```python
from build123d import *

# Parameters (mm, degrees)
SKETCH1_R               = 19.05
BOSS_EXTRUDE1_DEPTH     = 12.7
SKETCH2_R               = 3.175
BOSS_EXTRUDE2_DEPTH     = 12.7
CUT_EXTRUDE1_DEPTH      = 30.784140075
CUT_EXTRUDE1_DEPTH_BACK = 30.784140075
SKETCH4_R               = 6.477
SKETCH5_R               = 3.175
CUT_EXTRUDE2_DEPTH      = 73.66


with BuildPart() as part:
    # Sketch1 → Boss-Extrude1 (new body)
    with BuildSketch(Plane.XY):
        Circle(SKETCH1_R)
    extrude(amount=BOSS_EXTRUDE1_DEPTH)

    # Sketch2 → Boss-Extrude2 (add)
    with BuildSketch(Plane(origin=(0, 0, 0), x_dir=(-1, 0, 0), z_dir=(0, 0, -1))):
        with Locations(Location((0, 0, 0), (0, 0, 180))):
            Circle(SKETCH2_R)
    extrude(amount=BOSS_EXTRUDE2_DEPTH)

    # Sketch4 → Cut-Extrude1 (cut, two sides: drawn at the far end of the back side and taken through both)
    with BuildSketch(Plane(origin=(0, 0, 0), x_dir=(1, 0, 0), z_dir=(0, 1, 0)).offset(-CUT_EXTRUDE1_DEPTH_BACK)):
        with Locations((0, -12.7)):
            Circle(SKETCH4_R)
    extrude(amount=CUT_EXTRUDE1_DEPTH + CUT_EXTRUDE1_DEPTH_BACK, mode=Mode.SUBTRACT)

    # Sketch5 → Cut-Extrude2 (cut)
    with BuildSketch(Plane.XY.offset(12.7)):
        with Locations((12.7, 0)):
            Circle(SKETCH5_R)
        with Locations((-12.7, 0)):
            Circle(SKETCH5_R)
    extrude(amount=-CUT_EXTRUDE2_DEPTH, mode=Mode.SUBTRACT)


solid = part.part
```
Could you check a few things on this model? Use its own coordinates, in mm. Coordinates: 2 decimals unless noted, no trailing zeros. Write each loop counter-clockwise with the first axis right and the second up, starting at its lowest first coordinate (ties: lowest second). Pieces come first, ordered by that corner, then holes. Notation, with made-up numbers: (5.25, 32.5) -> (48.25, 32.5) arc R23 cw to (48.25, 46.5) -> close; hole circle Ø7 at (22, 30). An arc over 180 degrees is marked (long way). Return JSON: item names as keys, results as strings.
(1) Imagine slicing it at B-B, the plane x = 0. Please give me the cut outline in (y, z) (3 decimals).
Numbers:
{"outline": "(-19.05, 0) -> (-3.175, 0) -> (-3.175, -12.7) -> (3.175, -12.7) -> (3.175, 0) -> (19.05, 0) -> (19.05, 6.223) -> (-19.05, 6.223) -> close"}
(2) Imagine slicing it at D-D, the plane x = -13. Please give me the cut outline in (y, z).
Numbers:
{"outline": "(-13.92, 0) -> (-3.16, 0) -> (-3.16, 12.7) -> (-13.92, 12.7) -> close; (3.16, 0) -> (13.92, 0) -> (13.92, 12.7) -> (3.16, 12.7) -> close"}
(3) Imagine slicing it at C-C, the plane z = 9.5. Please give me the cut outline in (x, y) (3 decimals), then the cut area to 3 significant figures.
Numbers:
{"outline": "(-5.631, -18.199) -> (-5.631, 18.199) arc R19.05 ccw to start; (5.631, -18.199) arc R19.05 ccw to (5.631, 18.199) -> close; hole circle Ø6.35 at (-12.7, 0); hole circle Ø6.35 at (12.7, 0)", "area": "654 mm2"}
(4) I need wall thicknesses on L1, parallel to Y at x = -12.7, z = 10.25 (3 decimals); L2, parallel to Z at x = 7.5, y = 11.5; L3, parallel to Y at x = -12, z = 7.25. Which ranges of each line are inside material? Lowest first, please.
Numbers:
{"L1": "y = -14.199 to -3.175, 3.175 to 14.199", "L2": "z = 0 to 12.7", "L3": "y = -14.8 to -3.1, 3.1 to 14.8"}
(5) Imagine slicing it at A-A, the plane y = 0. Please give me the cut outline in (x, z) (3 decimals).
Numbers:
{"outline": "(-19.05, 0) -> (-15.875, 0) -> (-15.875, 12.7) -> (-19.05, 12.7) -> close; (-9.525, 0) -> (-3.175, 0) -> (-3.175, -12.7) -> (3.175, -12.7) -> (3.175, 0) -> (9.525, 0) -> (9.525, 12.7) -> (6.477, 12.7) arc R6.477 cw to (-6.477, 12.7) -> (-9.525, 12.7) -> close; (15.875, 0) -> (19.05, 0) -> (19.05, 12.7) -> (15.875, 12.7) -> close"}
(6) We'd pull the mould along X, two halves only. Please class faces 1 (the flat face through (0, 0, -12.7)), 2 (the cylindrical face through (-9.67, 0.95, 6.44)), 3 (the cylindrical face through (1.5, 2.8, -6.3)): +X half, -X half, draft (parallel to the pull), parting line (faces both ways), or undercut.
Numbers:
{"face 1": "draft", "face 2": "undercut", "face 3": "parting line"}
(7) I'm going to push flat-ended pins straight in: pin 1 (3 mm diameter, centred on y = -0.5, z = 3, fed in from +X); pin 2 (1 mm diameter, centred on x = -4.5, y = 7.5, fed in from -Z); pin 3 (8 mm diameter, centred on y = 7, z = 6, fed in from -X); pin 4 (4 mm diameter, centred on x = -4.5, z = -3, fed in from +Y). Where does each tip first touch, or does it pass through?
Numbers:
{"pin 1": "stops at x = 19.05", "pin 2": "stops at z = 0", "pin 3": "stops at x = -18.81", "pin 4": "stops at y = 1.96"}
